from build123d import *

# Parameters (mm, degrees)
SKETCH_1_R          = 10
EXTRUDE_1_DEPTH     = 20
SKETCH_2_R          = 45
EXTRUDE_2_DEPTH     = 20
CUT_EXTRUDE_1_DEPTH = 20
SKETCH_4_R          = 10
CUT_EXTRUDE_2_DEPTH = 10


with BuildPart() as part:
    # 草图1 → 凸台-拉伸1 (new body)
    with BuildSketch(Plane(origin=(0, 0, 0), x_dir=(0, 0, -1), z_dir=(1, 0, 0))):
        Circle(SKETCH_1_R)
    extrude(amount=EXTRUDE_1_DEPTH)

    # 草图2 → 凸台-拉伸2 (add)
    with BuildSketch(Plane(origin=(20, 0, 0), x_dir=(0, 0, -1), z_dir=(1, 0, 0))):
        Circle(SKETCH_2_R)
    extrude(amount=EXTRUDE_2_DEPTH)

    # 草图3 → 切除-拉伸1 (cut)
    with BuildSketch(Plane.ZY.offset(-20)):
        with BuildLine():
            Line((-9.705714191, 36.222218486), (-3.882285677, 14.488887394))
            ThreePointArc((-3.882285677, 14.488887394), (0, 15), (3.882285677, 14.488887394))
            Line((3.882285677, 14.488887394), (9.705714191, 36.222218486))
            ThreePointArc((9.705714191, 36.222218486), (0, 37.5), (-9.705714191, 36.222218486))
        make_face()
        with BuildLine():
            Line((26.516504294, 26.516504294), (10.606601718, 10.606601718))
            ThreePointArc((10.606601718, 10.606601718), (12.990381057, 7.5), (14.488887394, 3.882285677))
            Line((14.488887394, 3.882285677), (36.222218486, 9.705714191))
            ThreePointArc((36.222218486, 9.705714191), (32.475952642, 18.75), (26.516504294, 26.516504294))
        make_face()
        with BuildLine():
            Line((36.222218486, -9.705714191), (14.488887394, -3.882285677))
            ThreePointArc((14.488887394, -3.882285677), (12.990381057, -7.5), (10.606601718, -10.606601718))
            Line((10.606601718, -10.606601718), (26.516504294, -26.516504294))
            ThreePointArc((26.516504294, -26.516504294), (32.475952642, -18.75), (36.222218486, -9.705714191))
        make_face()
        with BuildLine():
            Line((9.705714191, -36.222218486), (3.882285677, -14.488887394))
            ThreePointArc((3.882285677, -14.488887394), (0, -15), (-3.882285677, -14.488887394))
            Line((-3.882285677, -14.488887394), (-9.705714191, -36.222218486))
            ThreePointArc((-9.705714191, -36.222218486), (0, -37.5), (9.705714191, -36.222218486))
        make_face()
        with BuildLine():
            Line((-26.516504294, -26.516504294), (-10.606601718, -10.606601718))
            ThreePointArc((-10.606601718, -10.606601718), (-12.990381057, -7.5), (-14.488887394, -3.882285677))
            Line((-14.488887394, -3.882285677), (-36.222218486, -9.705714191))
            ThreePointArc((-36.222218486, -9.705714191), (-32.475952642, -18.75), (-26.516504294, -26.516504294))
        make_face()
        with BuildLine():
            Line((-36.222218486, 9.705714191), (-14.488887394, 3.882285677))
            ThreePointArc((-14.488887394, 3.882285677), (-12.990381057, 7.5), (-10.606601718, 10.606601718))
            Line((-10.606601718, 10.606601718), (-26.516504294, 26.516504294))
            ThreePointArc((-26.516504294, 26.516504294), (-32.475952642, 18.75), (-36.222218486, 9.705714191))
        make_face()
    extrude(amount=-CUT_EXTRUDE_1_DEPTH, mode=Mode.SUBTRACT)

    # 草图4 → 切除-拉伸2 (cut)
    with BuildSketch(Plane(origin=(40, 0, 0), x_dir=(0, 0, -1), z_dir=(1, 0, 0))):
        Circle(SKETCH_4_R)
    extrude(amount=-CUT_EXTRUDE_2_DEPTH, mode=Mode.SUBTRACT)


solid = part.part
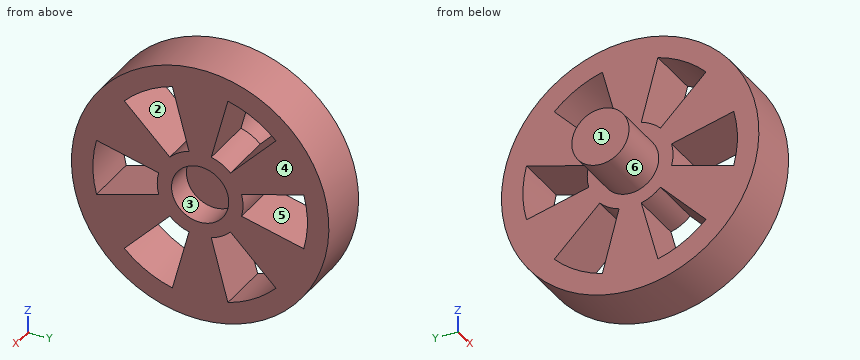
Verification items for the finished model (mm, model axes). Face numbers are marked on the shaded views. A direction names the side the tool comes from. Round coordinates to 2 decimals unless told otherwise and drop trailing zeros. Loops run counter-clockwise (first coordinate to the right, second up) from the corner with the lowest first, then second, coordinate; pieces in that order, holes last. Notation, with made-up numbers: M 68.5,-3 L 84.5,-3 A28 cw 84.5,35 Z; hole C -23.75,-31.75 d3. An arc over 180 degrees is marked long. Write each question's results on one line, items separated by ' | '.
1) Access from +Z, -Z, +X, -X, +Y, -Y to the whole of each face (thin tool, end or side, straight path). Record for the marked faces 1, 2 and 3.
Checks:
face 1: +Z, -Z, -X, +Y, -Y | face 2: +X, -X | face 3: +X
2) Mould release check, pull along Y, two halves, no side actions. Record for the marked faces 4, 5 and 6: released by +Y, released by -Y, zero draft, split by the parting line, or undercut.
Checks:
face 4: zero draft | face 5: undercut | face 6: split by the parting line
3) Gauge pin test, flat ends, axial feed: P1, Ø3, axis at x = 30, z = 27, coming from the -Y side; P2, Ø1, axis at y = -20.5, z = -15, coming from the -X side; P3, Ø8, axis at x = 25.5, z = -8, coming from the +Y side. Record the tip position at first contact, or that the pin passes through.
Checks:
P1: stops at y = -37.08 | P2: stops at x = 20 | P3: stops at y = 44.82
4) Section check D-D on x = 26. Record the boundary of the cut face in (y, z), then the cut area to 3 significant figures.
Checks:
outline: C 0,0 d90; hole M -36.22,-9.71 L -14.49,-3.88 A15 cw -14.49,3.88 L -36.22,9.71 A37.5 ccw Z; hole M -26.52,-26.52 A37.5 ccw -9.71,-36.22 L -3.88,-14.49 A15 cw -10.61,-10.61 Z; hole M -26.52,26.52 L -10.61,10.61 A15 cw -3.88,14.49 L -9.71,36.22 A37.5 ccw Z; hole M 3.88,-14.49 L 9.71,-36.22 A37.5 ccw 26.52,-26.52 L 10.61,-10.61 A15 cw Z; hole M 3.88,14.49 A15 cw 10.61,10.61 L 26.52,26.52 A37.5 ccw 9.71,36.22 Z; hole M 14.49,-3.88 L 36.22,-9.71 A37.5 ccw 36.22,9.71 L 14.49,3.88 A15 cw Z | area: 4,510 mm2
5) Section check A-A on z = 0. Record the boundary of the cut face in (x, y).
Checks:
outline: M 0,-10 L 20,-10 L 20,-15 L 40,-15 L 40,-10 L 30,-10 L 30,10 L 40,10 L 40,15 L 20,15 L 20,10 L 0,10 Z; M 20,-45 L 40,-45 L 40,-37.5 L 20,-37.5 Z; M 20,37.5 L 40,37.5 L 40,45 L 20,45 Z
6) Section check B-B on x = 35. Record the boundary of the cut face in (y, z).
Checks:
outline: C 0,0 d90; hole M -36.22,-9.71 L -14.49,-3.88 A15 cw -14.49,3.88 L -36.22,9.71 A37.5 ccw Z; hole M -26.52,-26.52 A37.5 ccw -9.71,-36.22 L -3.88,-14.49 A15 cw -10.61,-10.61 Z; hole M -26.52,26.52 L -10.61,10.61 A15 cw -3.88,14.49 L -9.71,36.22 A37.5 ccw Z; hole C 0,0 d20; hole M 3.88,-14.49 L 9.71,-36.22 A37.5 ccw 26.52,-26.52 L 10.61,-10.61 A15 cw Z; hole M 3.88,14.49 A15 cw 10.61,10.61 L 26.52,26.52 A37.5 ccw 9.71,36.22 Z; hole M 14.49,-3.88 L 36.22,-9.71 A37.5 ccw 36.22,9.71 L 14.49,3.88 A15 cw Z
7) Scan lines: L1, parallel to Y at x = 36, z = -19.5 (3 decimals); L2, parallel to Y at x = 33.5, z = -29; L3, parallel to Z at x = 20.5, y = 11. Record each from-to range of solid material in increasing order. Write a range as from..to.
Checks:
L1: y = -40.556..-19.5, -5.225..5.225, 19.5..40.556 | L2: y = -34.41..-23.77, -7.77..7.77, 23.77..34.41 | L3: z = -43.63..-35.85, -11..11, 35.85..43.63
8) Section check C-C on y = -24. Record the boundary of the cut face in (x, z).
Checks:
outline: M 20,-38.07 L 40,-38.07 L 40,-28.81 L 20,-28.81 Z; M 20,-24 L 40,-24 L 40,-6.43 L 20,-6.43 Z; M 20,6.43 L 40,6.43 L 40,24 L 20,24 Z; M 20,28.81 L 40,28.81 L 40,38.07 L 20,38.07 Z
